```python
from build123d import *

# Parameters (mm, degrees)
BOSS_EXTRUDE1_DEPTH = 1.5875
CUT_EXTRUDE1_DEPTH  = 303.12680487
CUT_EXTRUDE2_DEPTH  = 1.5875
FILLET1_R           = 5.08
SKETCH4_R           = 3.937
CUT_EXTRUDE3_DEPTH  = 303.056645934


with BuildPart() as part:
    # Sketch1 → Boss-Extrude1 (new body)
    with BuildSketch(Plane.XY):
        Polygon((-274.065317552, 28.949090055), (0, 0), (0, 116.332), (-278.827817552, 105.657090055), (-278.827817552, 88.385090055), (-278.827817552, 75.685090055), (-274.065317552, 75.685090055), align=None)
    extrude(amount=BOSS_EXTRUDE1_DEPTH)

    # Sketch2 → Cut-Extrude1 (cut, through all)
    with BuildSketch(Plane.XY.offset(1.5875)):
        Polygon((0, 116.332), (0, 65.532), (-4.7625, 65.532), (-4.7625, 116.14966791), align=None)
        Polygon((0, -5.469950558), (-4.7625, -5.469950558), (-4.7625, 0.503055413), (0, 0), align=None)
    extrude(amount=-CUT_EXTRUDE1_DEPTH, mode=Mode.SUBTRACT)

    # Sketch3 → Cut-Extrude2 (cut)
    with BuildSketch(Plane.XY.offset(1.5875)):
        Polygon((-240.657781537, 94.409124071), (-157.755224497, 97.583044587), (-203.185900054, 75.261166333), align=None)
        Polygon((-255.015317552, 87.483730445), (-255.015317552, 49.79533442), (-217.414707933, 68.269993226), align=None)
        Polygon((-248.210308368, 38.988718693), (-203.29748305, 61.056156751), (-137.156149504, 27.258241905), align=None)
        Polygon((-189.068675171, 68.047329858), (-136.005712706, 94.119250944), (-90.836715855, 62.962907236), (-131.496140727, 38.628031633), align=None)
        Polygon((-120.716079793, 99.001086509), (-24.466190753, 102.686009006), (-78.860877706, 70.130508168), align=None)
        Polygon((-127.472455762, 26.235368508), (-79.347844483, 55.0381967), (-21.337942125, 15.024546137), align=None)
        Polygon((-67.372006334, 62.205797632), (-23.8125, 88.276386956), (-23.8125, 32.159636644), align=None)
    extrude(amount=-CUT_EXTRUDE2_DEPTH, mode=Mode.SUBTRACT)

    # Fillet1
    fillet1_edges = [part.edges().sort_by_distance(p)[0] for p in [
        (-255.015317552, 87.483730445, 0.79375),
        (-217.414707933, 68.269993226, 0.79375),
        (-255.015317552, 49.79533442, 0.79375),
        (-127.472455762, 26.235368508, 0.79375),
        (-21.337942125, 15.024546137, 0.79375),
        (-79.347844483, 55.0381967, 0.79375),
        (-248.210308368, 38.988718693, 0.79375),
        (-137.156149504, 27.258241905, 0.79375),
        (-203.29748305, 61.056156751, 0.79375),
        (-240.657781537, 94.409124071, 0.79375),
        (-203.185900054, 75.261166333, 0.79375),
        (-157.755224497, 97.583044587, 0.79375),
        (-136.005712706, 94.119250944, 0.79375),
        (-189.068675171, 68.047329858, 0.79375),
        (-131.496140727, 38.628031633, 0.79375),
        (-90.836715855, 62.962907236, 0.79375),
        (-67.372006334, 62.205797632, 0.79375),
        (-23.8125, 32.159636644, 0.79375),
        (-23.8125, 88.276386956, 0.79375),
        (-24.466190753, 102.686009006, 0.79375),
        (-120.716079793, 99.001086509, 0.79375),
        (-78.860877706, 70.130508168, 0.79375),
    ]]
    fillet(fillet1_edges, radius=FILLET1_R)

    # Sketch4 → Cut-Extrude3 (cut, through all)
    with BuildSketch(Plane.XY.offset(1.5875)):
        with Locations((-253.745317552, 39.57337304)):
            Circle(SKETCH4_R)
    extrude(amount=-CUT_EXTRUDE3_DEPTH, mode=Mode.SUBTRACT)


solid = part.part
```
Could you check a few things on this model? Use its own coordinates, in mm. A direction names the side the tool comes from. Round coordinates to 2 decimals unless told otherwise and drop trailing zeros. Loops run counter-clockwise (first coordinate to the right, second up) from the corner with the lowest first, then second, coordinate; pieces in that order, holes last. Notation, with made-up numbers: M 80.25,29 L 124.25,29 A31 ccw 124.25,67 Z; hole C -9,50.25 d5. An arc over 180 degrees is marked long. Put each result on its own line as item: value.
Q1. Imagine slicing it at A-A (x = -167). Write out the boundary of the cut face in (y, z).
Check result:
outline: M 17.64,0 L 30.41,0 L 30.41,1.59 L 17.64,1.59 Z; M 42.51,0 L 56.77,0 L 56.77,1.59 L 42.51,1.59 Z; M 78.89,0 L 109.94,0 L 109.94,1.59 L 78.89,1.59 Z
Q2. For pin 1 (0.8 mm diameter, centred on x = -277.5, z = 0.5, fed in from -Y); pin 2 (0.8 mm diameter, centred on y = 101.5, z = 0.5, fed in from +X); pin 3 (0.5 mm diameter, centred on y = 46.5, z = 1, fed in from -X); pin 4 (9 mm diameter, centred on x = -253.75, y = 39.57, fed in from -Z), each with a flat end and sliding along its axis, tell me the tip position at first contact or that it passes through.
Check result:
pin 1: y = 75.69
pin 2: x = -4.76
pin 3: x = -274.07
pin 4: z = 0
Q3. Imagine slicing it at B-B (x = -239). Write out the boundary of the cut face in (y, z), then the cut area to 3 significant figures.
Check result:
outline: M 25.25,0 L 57.66,0 L 57.66,1.59 L 25.25,1.59 Z; M 79.3,0 L 107.18,0 L 107.18,1.59 L 79.3,1.59 Z
area: 95.7 mm2
Q4. I need wall thicknesses on probe 1 along Y at (x, z) = (-88.5, 0.95); probe 2 along X at (y, z) = (82, 0.9); probe 3 along X at (y, z) = (81.5, 0.45). Which ranges of each line are inside material? Lowest first, please.
Check result:
probe 1: 9.35 to 22.12, 49.56 to 76.78, 100.23 to 112.94
probe 2: -278.83 to -254.16, -244.28 to -216.37, -189.47 to -160.67, -118.44 to -96.07, -59.03 to -34.3, -24.58 to -4.76
probe 3: -278.83 to -254.46, -243.31 to -215.4, -190.49 to -161.69, -117.71 to -95.34, -59.86 to -35.13, -24.31 to -4.76
Q5. On a 3-axis mill with a long thin cutter (end or side, diameter ignored), from which of +Z, -Z, +X, -X, +Y, -Y can I reach the whole of each face in a straight line? I mean faces 4 (the face through (-26.322, 83.697, 0.783)), 5 (the face through (-110, 46, 0)). Say none if no direction works.
Check result:
face 4: +Z, -Z
face 5: -Z, +X, -X, +Y, -Y
Q6. Imagine slicing it at D-D (z = 0.6). State how many separate pieces and enclosed holes the cut face has, then the cut area to 3 significant figures.
Check result:
separate pieces: 1
enclosed holes: 8
area: 16,800 mm2
Q7. Imagine slicing it at C-C (x = -208.5). Write out the boundary of the cut face in (y, z), then the cut area to 3 significant figures.
Check result:
outline: M 22.02,0 L 34.79,0 L 34.79,1.59 L 22.02,1.59 Z; M 58.5,0 L 77.98,0 L 77.98,1.59 L 58.5,1.59 Z; M 95.64,0 L 108.35,0 L 108.35,1.59 L 95.64,1.59 Z
area: 71.4 mm2
Q8. Thinking about a two-plate mould opening in Y: for faces 1 (the face through (-35.917, 20.321, 0.783)), 2 (the face through (-139.877, 110.977, 0.783)), 3 (the face through (-138.951, 14.677, 0.783)), which applies, released by +Y, released by -Y, zero draft, split by the parting line, or undercut?
Check result:
face 1: undercut
face 2: released by +Y
face 3: released by -Y
